Can you work these out from the model? Positions are in its coordinate system, mm. Give positions to 0.01 mm unless a question says otherwise; leave off trailing zeros. Write each loop counter-clockwise with the first axis right and the second up, starting at its lowest first coordinate (ties: lowest second). Pieces come first, ordered by that corner, then holes. Notation, with made-up numbers: (44.5, 47) -> (86.5, 47) arc R23 cw to (86.5, 63) -> close; hole circle Ø5 at (83, -15.75). An arc over 180 degrees is marked (long way). Answer as CSV lines item,"result". Start each with the question number.
1. If we section it at D-D on x = 4: Write out the boundary of the cut face in (y, z), plus the area to 3 significant figures.
2. If we section it at C-C on z = 0.75: Write out the boundary of the cut face in (x, y).
3. If we section it at A-A on y = -57: Write out the boundary of the cut face in (x, z).
4. I need wall thicknesses on line 1 (Y direction, x = -8.5, z = 2); line 2 (X direction, y = 42.5, z = 2.35); line 3 (Y direction, x = -11.5, z = 0.7). Which ranges of each line are inside material? Lowest first, please. Write a range as [from, to].
5. I'm going to push flat-ended pins straight in: P1, Ø2, axis at x = 8.5, y = -57, coming from the -Z side; P2, Ø1.5, axis at x = -11.5, z = 2, coming from the +Y side. Where does each tip first touch, or does it pass through?
6. If we section it at B-B on x = -8.5: Write out the boundary of the cut face in (y, z).
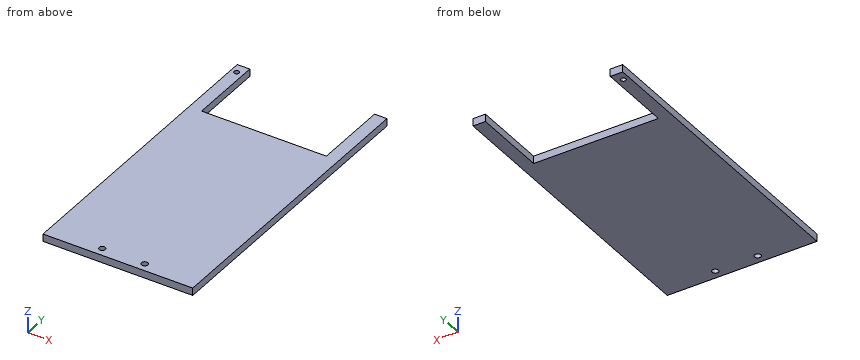
```python
from build123d import *

# Parameters (mm, degrees)
F1_DEPTH = 2
F2_R     = 1
F3_DEPTH = 25
F4_DEPTH = 3
F6_R     = 1.25
F7_DEPTH = 5
F5_R     = 1
F8_DEPTH = 25


with BuildPart() as f1:
    # F0 (on Top) → F1 (new body)
    with BuildSketch(Plane.XY):
        Polygon((-25, 60.5), (-30, 60.5), (-30, -60.5), (30, -60.5), (30, 60.5), (25, 60.5), (25, 30.5), (-25, 30.5), align=None)
    extrude(amount=F1_DEPTH)

    # F2 (on face) → F3 (cut)
    with BuildSketch(Plane.XY.offset(2)):
        with Locations((-27.5, 57)):
            Circle(F2_R)
    extrude(amount=-F3_DEPTH, mode=Mode.SUBTRACT)

    # F0 (on Top) → F4 (join)
    with BuildSketch(Plane.XY):
        Polygon((-25, 60.5), (-30, 60.5), (-30, -60.5), (30, -60.5), (30, 60.5), (25, 60.5), (25, 30.5), (-25, 30.5), align=None)
    extrude(amount=F4_DEPTH)

    # F6 (on face) → F7 (cut)
    with BuildSketch(Plane.XY.offset(3)):
        with Locations((-8.5, -57)):
            Circle(F6_R)
        with Locations((8.5, -57)):
            Circle(F6_R)
    extrude(amount=-F7_DEPTH, mode=Mode.SUBTRACT)

    # F5 (on face) → F8 (cut)
    with BuildSketch(Plane.XY.offset(3)):
        with Locations((-27.689109, 56.5)):
            Circle(F5_R)
    extrude(amount=-F8_DEPTH, mode=Mode.SUBTRACT)


solid = f1.part
```
Computed values:
1,outline,"(-60.5, 0) -> (30.5, 0) -> (30.5, 3) -> (-60.5, 3) -> close"
1,area,"273 mm2"
2,outline,"(-30, -60.5) -> (30, -60.5) -> (30, 60.5) -> (25, 60.5) -> (25, 30.5) -> (-25, 30.5) -> (-25, 60.5) -> (-30, 60.5) -> close; hole circle Ø2 at (-27.69, 56.5); hole circle Ø2.5 at (-8.5, -57); hole circle Ø2.5 at (8.5, -57)"
3,outline,"(-30, 0) -> (-9.75, 0) -> (-9.75, 3) -> (-30, 3) -> close; (-7.25, 0) -> (7.25, 0) -> (7.25, 3) -> (-7.25, 3) -> close; (9.75, 0) -> (30, 0) -> (30, 3) -> (9.75, 3) -> close"
4,line 1,"y = [-60.5, -58.25], [-55.75, 30.5]"
4,line 2,"x = [-30, -25], [25, 30]"
4,line 3,"y = [-60.5, 30.5]"
5,P1,"passes through"
5,P2,"stops at y = 30.5"
6,outline,"(-60.5, 0) -> (-58.25, 0) -> (-58.25, 3) -> (-60.5, 3) -> close; (-55.75, 0) -> (30.5, 0) -> (30.5, 3) -> (-55.75, 3) -> close"
